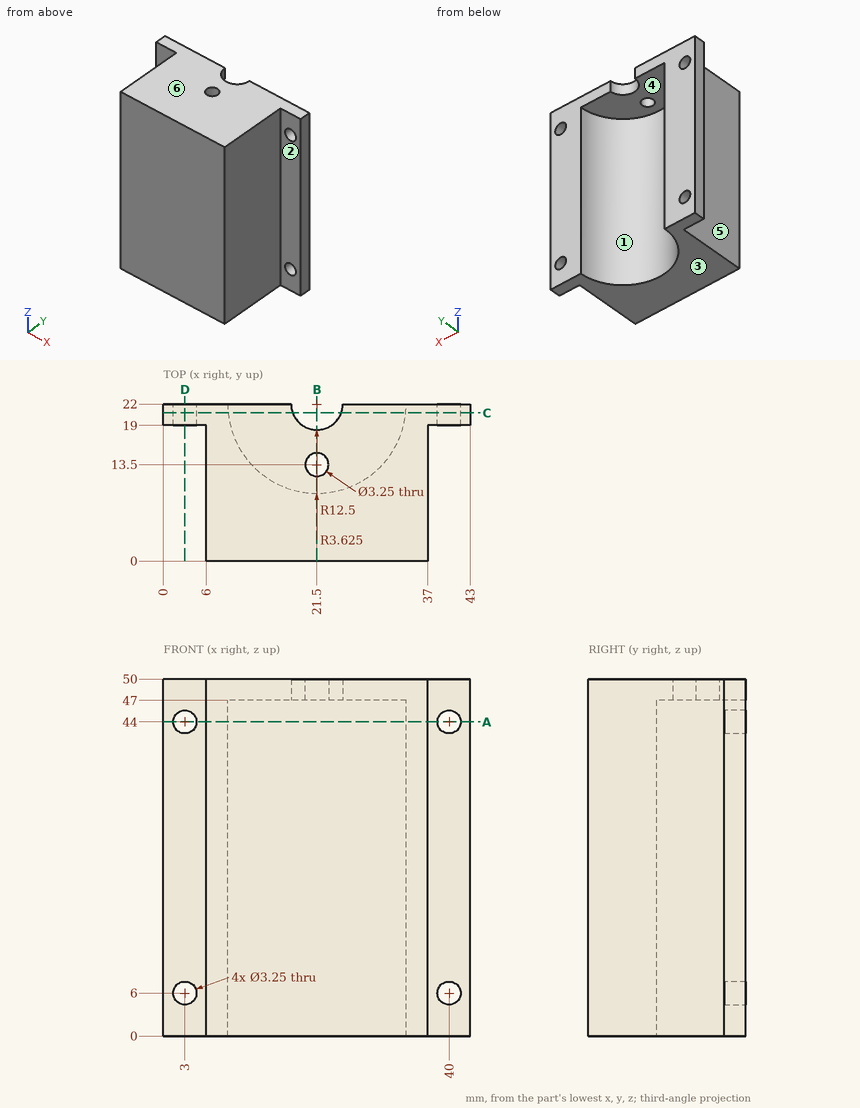
Verification items for this drawing (mm, ordinates from the low corner). A direction names the side the tool comes from. Round coordinates to 2 decimals unless told otherwise and drop trailing zeros. Order: outer loops, then holes, each group sorted by start corner. A loop starts at its lowest first (then second) coordinate and runs counter-clockwise, first axis right, second up. Notation, with made-up numbers: (-35.5, -32.75) - (-7.5, -32.75) arc R36 ccw to (-7.5, 2.25) - close; hole circle Ø8 at (29, 34.25). An arc over 180 degrees is marked (long way). Answer as CSV lines item,"result". Start each with the question number.
1) Scan lines: probe 1 along X at (y, z) = (20.55, 44) (3 decimals); probe 2 along Y at (x, z) = (41, 12.5); probe 3 along Z at (x, y) = (17, 13). Record each from-to range of solid material in increasing order.
2) Tool access check on the marked faces 1, 2 and 3. Record the directions out of +Z, -Z, +X, -X, +Y, -Y that give a thin tool (end or side, any length) a straight path to the whole face; none if there is none.
3) Section check C-C (y = 20.75). Record the cut outline in (x, z) (3 decimals).
4) Section check D-D (x = 3). Record the cut outline in (y, z) (3 decimals), then the cut area to 4 significant figures.
5) Section check A-A (z = 44). Record the cut outline in (x, y) (3 decimals).
6) Section check B-B (x = 21.5). Record the cut outline in (y, z) (3 decimals).
7) Depth check by flat-ended pin: pin 1 (1.5 mm diameter, centred on x = 19, z = 7.5, fed in from +Y); pin 2 (12 mm diameter, centred on x = 28.5, z = 35, fed in from -Y); pin 3 (4 mm diameter, centred on x = 29.5, z = 20, fed in from +Y); pin 4 (4 mm diameter, centred on x = 23.5, y = 18.5, fed in from -Z). Enter the tip coordinate at first touch or a pass-through.
8) Draft check along X on the marked faces 4, 5 and 6. Enter one of: +X half, -X half, draft (parallel to the pull), parting line (faces both ways), or undercut.
Determined:
1,probe 1,"0 to 1.375, 4.625 to 9.084, 33.916 to 38.375, 41.625 to 43"
1,probe 2,"19 to 22"
1,probe 3,"47 to 50"
2,face 1,"-Z, +Y"
2,face 2,"+Z, -Z, +X, -Y"
2,face 3,"-Z, +X, -X, +Y, -Y"
3,outline,"(0, 0) - (9.063, 0) - (9.063, 47) - (18.097, 47) - (18.097, 50) - (0, 50) - close; (24.903, 47) - (33.937, 47) - (33.937, 0) - (43, 0) - (43, 50) - (24.903, 50) - close; hole circle Ø3.25 at (3, 6); hole circle Ø3.25 at (3, 44); hole circle Ø3.25 at (40, 6); hole circle Ø3.25 at (40, 44)"
4,outline,"(19, 0) - (22, 0) - (22, 4.375) - (19, 4.375) - close; (19, 7.625) - (22, 7.625) - (22, 42.375) - (19, 42.375) - close; (19, 45.625) - (22, 45.625) - (22, 50) - (19, 50) - close"
4,area,"130.5 mm^2"
5,outline,"(0, 19) - (1.375, 19) - (1.375, 22) - (0, 22) - close; (4.625, 19) - (6, 19) - (6, 0) - (37, 0) - (37, 19) - (38.375, 19) - (38.375, 22) - (34, 22) arc R12.5 cw to (9, 22) - (4.625, 22) - close; (41.625, 19) - (43, 19) - (43, 22) - (41.625, 22) - close"
6,outline,"(0, 0) - (9.5, 0) - (9.5, 47) - (11.875, 47) - (11.875, 50) - (0, 50) - close; (15.125, 47) - (18.375, 47) - (18.375, 50) - (15.125, 50) - close"
7,pin 1,"y = 9.93"
7,pin 2,"y = 0"
7,pin 3,"y = 14.5"
7,pin 4,"z = 47"
8,face 4,"undercut"
8,face 5,"-X half"
8,face 6,"draft"
